The model under review builds one solid part; all positions refer to its coordinate system, in mm. A direction names the side the tool comes from. Give positions to 0.01 mm unless a question says otherwise; leave off trailing zeros. Loops run counter-clockwise (first coordinate to the right, second up) from the corner with the lowest first, then second, coordinate; pieces in that order, holes last. Notation, with made-up numbers: M -20.75,-3 L 13.25,-3 A25 ccw 13.25,22 Z; hole C 7.25,80.5 d10. An arc over 180 degrees is marked long. Return JSON: item names as keys, results as strings.
```python
from build123d import *

# Parameters (mm, degrees)
F0_W     = 47.7
F0_H     = 31.6
F1_DEPTH = 9.6
F2_W     = 45.3
F2_H     = 29.2
F3_DEPTH = 8.6
F4_R     = 2.4
F5_DEPTH = 1.8
F7_R     = 1.3
F8_DEPTH = 1.2


with BuildPart() as f1:
    # F0 (on Top) → F1 (new body)
    with BuildSketch(Plane.XY):
        Rectangle(F0_W, F0_H)
    extrude(amount=F1_DEPTH)

    # F2 (on face) → F3 (cut)
    with BuildSketch(Plane.XY):
        Rectangle(F2_W, F2_H)
    extrude(amount=F3_DEPTH, mode=Mode.SUBTRACT)

    # F4 (on face) → F5 (join)
    with BuildSketch(Plane.XY.offset(9.6)):
        with Locations((-19.9, 11.85)):
            Circle(F4_R)
        with Locations((-19.9, 3.85)):
            Circle(F4_R)
        with Locations((-19.9, -4.15)):
            Circle(F4_R)
        with Locations((-19.9, -12.15)):
            Circle(F4_R)
        with Locations((-11.9, 11.85)):
            Circle(F4_R)
        with Locations((-11.9, 3.85)):
            Circle(F4_R)
        with Locations((-11.9, -4.15)):
            Circle(F4_R)
        with Locations((-11.9, -12.15)):
            Circle(F4_R)
        with Locations((-3.9, 11.85)):
            Circle(F4_R)
        with Locations((-3.9, 3.85)):
            Circle(F4_R)
        with Locations((-3.9, -4.15)):
            Circle(F4_R)
        with Locations((-3.9, -12.15)):
            Circle(F4_R)
        with Locations((4.1, 11.85)):
            Circle(F4_R)
        with Locations((4.1, 3.85)):
            Circle(F4_R)
        with Locations((4.1, -4.15)):
            Circle(F4_R)
        with Locations((4.1, -12.15)):
            Circle(F4_R)
        with Locations((12.1, 11.85)):
            Circle(F4_R)
        with Locations((12.1, 3.85)):
            Circle(F4_R)
        with Locations((12.1, -4.15)):
            Circle(F4_R)
        with Locations((12.1, -12.15)):
            Circle(F4_R)
        with Locations((20.1, 11.85)):
            Circle(F4_R)
        with Locations((20.1, 3.85)):
            Circle(F4_R)
        with Locations((20.1, -4.15)):
            Circle(F4_R)
        with Locations((20.1, -12.15)):
            Circle(F4_R)
    extrude(amount=F5_DEPTH)

    # F7 (on offset) → F8 (cut)
    with BuildSketch(Plane.XY.offset(8.4)):
        with Locations((-19.9, -12.15)):
            Circle(F7_R)
        with Locations((-19.9, -4.15)):
            Circle(F7_R)
        with Locations((-19.9, 3.85)):
            Circle(F7_R)
        with Locations((-19.9, 11.85)):
            Circle(F7_R)
        with Locations((-11.9, -12.15)):
            Circle(F7_R)
        with Locations((-11.9, -4.15)):
            Circle(F7_R)
        with Locations((-11.9, 3.85)):
            Circle(F7_R)
        with Locations((-11.9, 11.85)):
            Circle(F7_R)
        with Locations((-3.9, -12.15)):
            Circle(F7_R)
        with Locations((-3.9, -4.15)):
            Circle(F7_R)
        with Locations((-3.9, 3.85)):
            Circle(F7_R)
        with Locations((-3.9, 11.85)):
            Circle(F7_R)
        with Locations((4.1, -12.15)):
            Circle(F7_R)
        with Locations((4.1, -4.15)):
            Circle(F7_R)
        with Locations((4.1, 3.85)):
            Circle(F7_R)
        with Locations((4.1, 11.85)):
            Circle(F7_R)
        with Locations((12.1, -12.15)):
            Circle(F7_R)
        with Locations((12.1, -4.15)):
            Circle(F7_R)
        with Locations((12.1, 3.85)):
            Circle(F7_R)
        with Locations((12.1, 11.85)):
            Circle(F7_R)
        with Locations((20.1, -12.15)):
            Circle(F7_R)
        with Locations((20.1, -4.15)):
            Circle(F7_R)
        with Locations((20.1, 3.85)):
            Circle(F7_R)
        with Locations((20.1, 11.85)):
            Circle(F7_R)
    extrude(amount=F8_DEPTH, mode=Mode.SUBTRACT)


solid = f1.part
```
1) Insertion check: pin 1 (5 mm diameter, centred on x = 5.5, y = -10.5, fed in from -Z); pin 2 (1.3 mm diameter, centred on x = 12.5, y = 12, fed in from -Z); pin 3 (6 mm diameter, centred on x = 13, z = 10, fed in from -Y). Each pin has a flat end and moves straight along its axis. Give the tip position at first contact, or say it passes through.
From the geometry:
{"pin 1": "z = 8.6", "pin 2": "z = 9.6", "pin 3": "y = -15.8"}
2) Consider section B-B on y = 7. Write out the cut boundary in (x, z).
From the geometry:
{"outline": "M -23.85,0 L -22.65,0 L -22.65,8.6 L 22.65,8.6 L 22.65,0 L 23.85,0 L 23.85,9.6 L -23.85,9.6 Z"}
3) Tool access review of faces 5 (the face through (-11.3, -13.303, 9.093)), 6 (the face through (-13.805, -5.61, 10.487)), 7 (the face through (-20, -12, 11.4)): name each direction out of +Z, -Z, +X, -X, +Y, -Y from which nothing blocks a thin tool from reaching the whole face with its end or side.
From the geometry:
{"face 5": "-Z", "face 6": "+Z", "face 7": "+Z, +X, -X, +Y, -Y"}
4) The part is to be moulded in two halves that separate along X. For faces 1 (the face through (14.317, 10.931, 10.487)), 2 (the face through (-23.85, 0, 5)), 3 (the face through (19.82, -13.42, 9.09)), 4 (the face through (12, -4, 11.4)), say which applies: released by +X, released by -X, zero draft, split by the parting line, or undercut.
From the geometry:
{"face 1": "undercut", "face 2": "released by -X", "face 3": "undercut", "face 4": "zero draft"}
5) Wall thickness on L1, parallel to Y at x = -19.9, z = 9.25; L2, parallel to X at y = 7.5, z = 5.5; L3, parallel to Y at x = 18.5, z = 3.5: over which ranges is each line inside the solid? List them lowest first. Write a range as from..to.
From the geometry:
{"L1": "-15.8..-13.45, -10.85..-5.45, -2.85..2.55, 5.15..10.55, 13.15..15.8", "L2": "-23.85..-22.65, 22.65..23.85", "L3": "-15.8..-14.6, 14.6..15.8"}
6) Consider section C-C on z = 5.25. Write out the cut boundary in (x, y).
From the geometry:
{"outline": "M -23.85,-15.8 L 23.85,-15.8 L 23.85,15.8 L -23.85,15.8 Z; hole M -22.65,-14.6 L 22.65,-14.6 L 22.65,14.6 L -22.65,14.6 Z"}
7) Consider section A-A on x = -0.5. Write out the cut boundary in (y, z), then the cut area to 3 significant figures.
From the geometry:
{"outline": "M -15.8,0 L -14.6,0 L -14.6,8.6 L 14.6,8.6 L 14.6,0 L 15.8,0 L 15.8,9.6 L -15.8,9.6 Z", "area": "52.2 mm²"}
